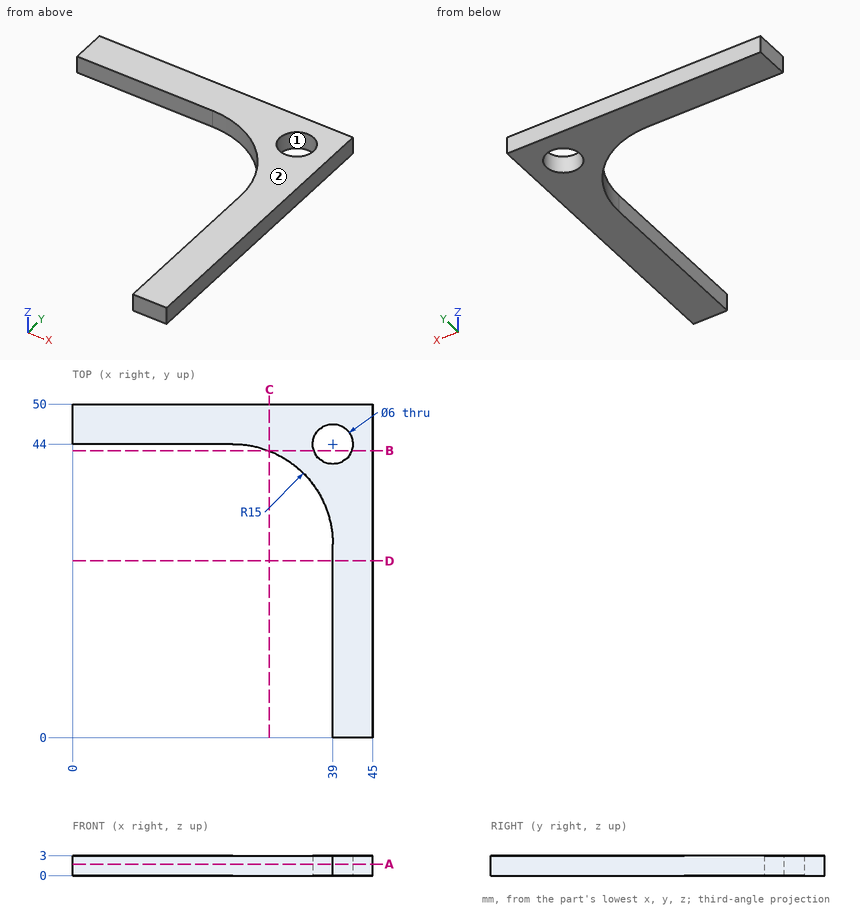
Check sheet for the drawn part. Datum: minimum x, y, z corner. Units: mm. Coordinates: 2 decimals unless noted, no trailing zeros. Order: outer loops, then holes, each group sorted by start corner. A loop starts at its lowest first (then second) coordinate and runs counter-clockwise, first axis right, second up. Notation, with made-up numbers: M 6,37 L 39,37 A31 cw 39,74 Z; hole C -34,-25 d11. An arc over 180 degrees is marked long. One line per question, with ' | ' between items. Start each with the question number.
Item 1: Material ranges on line 1 (X direction, y = 4, z = 1.2); line 2 (Y direction, x = 11, z = 2.75); line 3 (Y direction, x = 35.5, z = 0.2), recorded low to high.
Item 2: Sectioned sample at D-D on y = 26.5. Record the cut outline in (x, z), and give its area (3 significant figures).
Item 3: Sectioned sample at C-C on x = 29.5. Record the cut outline in (y, z).
Item 4: Sectioned sample at B-B on y = 43. Record the cut outline in (x, z), and give its area (3 significant figures).
Item 5: Sectioned sample at A-A on z = 1.75. Record the cut outline in (x, y).
Item 6: Gauge pin test, flat ends, axial feed: P1, Ø0.9, axis at x = 6.5, z = 1, coming from the -Y side; P2, Ø1, axis at y = 27.5, z = 2.5, coming from the -X side; P3, Ø1.5, axis at x = 31.5, z = 2, coming from the -Y side. Record the tip position at first contact, or that the pin passes through.
Item 7: Mould release check, pull along Y, two halves, no side actions. Record for the marked faces 1 and 2: pulls with the +Y half, pulls with the -Y half, needs draft (parallel to the pull), parting line crosses it, or undercut.
Answer below:
1) line 1: x = 39 to 45 | line 2: y = 44 to 50 | line 3: y = 38.63 to 50
2) outline: M 39,0 L 45,0 L 45,3 L 39,3 Z | area: 18.0 mm^2
3) outline: M 42.96,0 L 50,0 L 50,3 L 42.96,3 Z
4) outline: M 29.39,0 L 36.17,0 L 36.17,3 L 29.39,3 Z; M 41.83,0 L 45,0 L 45,3 L 41.83,3 Z | area: 29.9 mm^2
5) outline: M 0,44 L 24,44 A15 cw 39,29 L 39,0 L 45,0 L 45,50 L 0,50 Z; hole C 39,44 d6
6) P1: stops at y = 44 | P2: stops at x = 39 | P3: stops at y = 41.53
7) face 1: undercut | face 2: needs draft
